For this review, use the dimensioned drawing (mm, ordinates from the lowest corner) and the shaded views. A direction names the side the tool comes from. Round coordinates to 2 decimals unless told otherwise and drop trailing zeros. Loops run counter-clockwise (first coordinate to the right, second up) from the corner with the lowest first, then second, coordinate; pieces in that order, holes last.
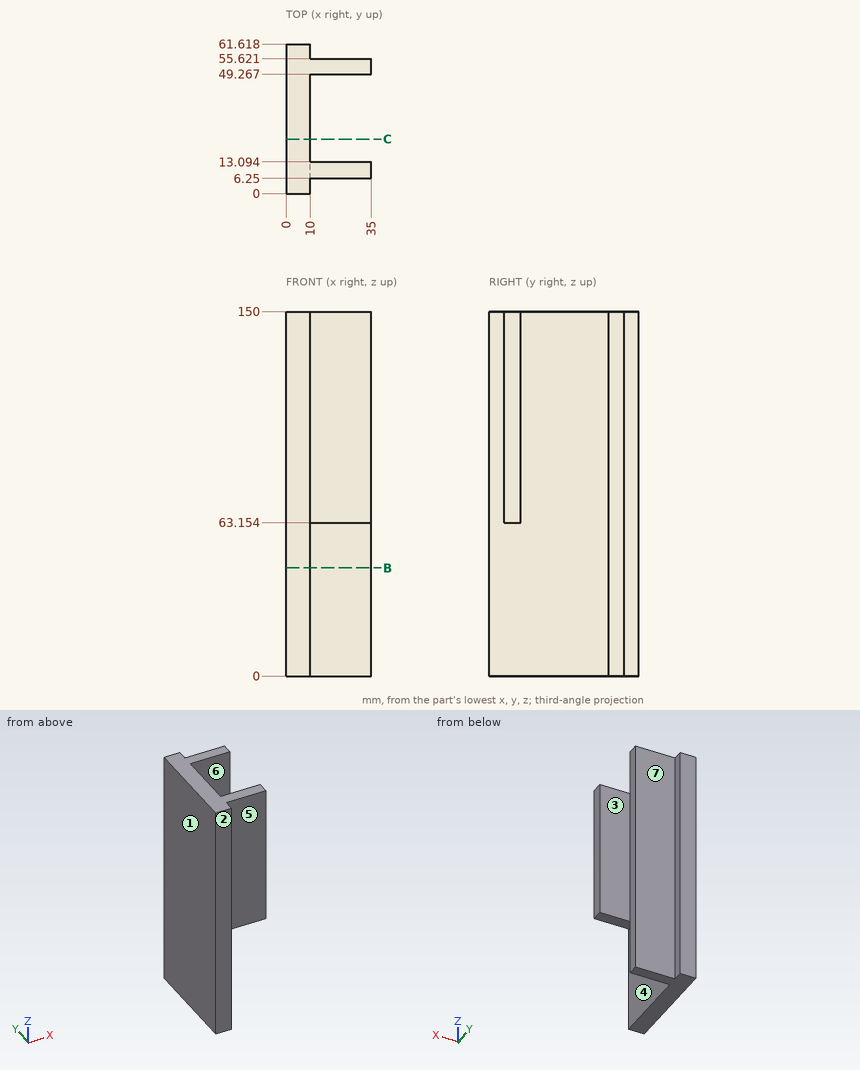
(1) Insertion check: pin 1 Ø8 at (x, z) = (21, 64.5) entering from +Y; pin 2 Ø3 at (y, z) = (59, 67) entering from +X; pin 3 Ø7.5 at (x, z) = (26.5, 88) entering from -Y. Each pin has a flat end and moves straight along its axis. Give the tip position at first contact, or say it passes through.
(2) For the marked faces 5, 6 and 7, list the 3-axis set-ups (+Z, -Z, +X, -X, +Y, -Y) from which the entire face can be reached by the end or side of a thin tool; tool diameter is ignored.
(3) Add section B-B (z = 44.5). Give the boundary of the cut face in (x, y).
(4) Add section C-C (y = 22.5). Give the boundary of the cut face in (x, z), plus the area to 3 significant figures.
(5) For L1, parallel to Y at x = 23, z = 79.5; L2, parallel to X at y = 46, z = 32; L3, parallel to Z at x = 29.5, y = 8 (1 decimal), list the stretches that pass through material, from the lowest coordinate up.
(6) The part is to be moulded in two halves that separate along Y. For the marked faces 1, 2, 3 and 4, say which applies: pulls with the +Y half, pulls with the -Y half, needs draft (parallel to the pull), parting line crosses it, or undercut.
Outcome:
1. pin 1: stops at y = 55.62
1. pin 2: stops at x = 10
1. pin 3: stops at y = 6.25
2. face 5: +Z, -Z, +X, -Y
2. face 6: +Z, -Z, +X
2. face 7: +Z, -Z, +X, +Y
3. outline: (0, 0) - (10, 0) - (10, 49.27) - (35, 49.27) - (35, 55.62) - (10, 55.62) - (10, 61.62) - (0, 61.62) - close
4. outline: (0, 0) - (10, 0) - (10, 150) - (0, 150) - close
4. area: 1,500 mm2
5. L1: y = 6.25 to 13.09, 49.27 to 55.62
5. L2: x = 0 to 10
5. L3: z = 63.2 to 150
6. face 1: needs draft
6. face 2: pulls with the -Y half
6. face 3: undercut
6. face 4: undercut
